from build123d import *

# Parameters (mm, degrees)
F2_R    = 1
F3_SIZE = 1


with BuildPart() as f1:
    # F0 (on Right) → F1 (revolve)
    with BuildSketch(Plane.YZ):
        Polygon((2.5, 27), (2.5, 0), (7.5, 0), (7.5, 30), (4, 30), (4, 50), (1.5, 50), (1.5, 27), align=None)
    revolve(axis=Axis((0, 0, 12.798217), (0, 0, -1)))

    # F2
    f2_edges = [f1.edges().sort_by_distance(p)[0] for p in [
        (0, -4, 50),
        (0, -4, 30),
        (0, -7.5, 30),
    ]]
    fillet(f2_edges, radius=F2_R)

    # F3
    f3_edges = [f1.edges().sort_by_distance(p)[0] for p in [
        (0, -7.5, 0),
    ]]
    chamfer(f3_edges, length=F3_SIZE)


solid = f1.part
The model under review builds one solid part; all positions refer to its coordinate system, in mm. A direction names the side the tool comes from. Give positions to 0.01 mm unless a question says otherwise; leave off trailing zeros. Write each loop counter-clockwise with the first axis right and the second up, starting at its lowest first coordinate (ties: lowest second). Pieces come first, ordered by that corner, then holes.
1. Tool access review of faces 1 (the flat face through (-1.3, 1.3, 50)), 2 (the flat face through (-5, 2, 30)): name each direction out of +Z, -Z, +X, -X, +Y, -Y from which nothing blocks a thin tool from reaching the whole face with its end or side.
2. Add section A-A, the plane y = 0. Write out the cut boundary in (x, z), plus the area to 3 significant figures.
3. Draft analysis for pull direction Y (two halves, no side actions). For faces 3 (the cylindrical face through (0.33, -7.493, 15.196)), 4 (the flat face through (0, -3, 0)), 5 (the flat face through (0, -2, 27)), 6 (the cylindrical face through (-2.44, -0.54, 13.31)), state which applies: +Y half, -Y half, draft (parallel to the pull), parting line (faces both ways), or undercut.
4. Wall thickness on L1, parallel to X at y = 0, z = 19.5; L2, parallel to X at y = 0, z = 33; L3, parallel to Y at x = -1.5, z = 26.5: over which ranges is each line inside the solid? List them lowest first.
5. For P1, Ø3, axis at x = -6, y = -4, coming from the -Z side; P2, Ø1, axis at y = 3.5, z = 42.5, coming from the -X side; P3, Ø3, axis at y = -5, z = 35.5, coming from the -X side; P4, Ø5, axis at x = -4.5, y = 5.5, coming from the +Z side, all flat-tipped, find the tip position at first contact; note any pin that passes through.
Worked answers:
1. face 1: +Z, +X, -X, +Y, -Y
1. face 2: +Z
2. outline: (-7.5, 1) - (-6.5, 0) - (-2.5, 0) - (-2.5, 27) - (-1.5, 27) - (-1.5, 50) - (-3, 50) arc R1 ccw to (-4, 49) - (-4, 31) arc R1 cw to (-5, 30) - (-6.5, 30) arc R1 ccw to (-7.5, 29) - close; (1.5, 27) - (2.5, 27) - (2.5, 0) - (6.5, 0) - (7.5, 1) - (7.5, 29) arc R1 ccw to (6.5, 30) - (5, 30) arc R1 cw to (4, 31) - (4, 49) arc R1 ccw to (3, 50) - (1.5, 50) - close
2. area: 405 mm2
3. face 3: parting line
3. face 4: draft
3. face 5: undercut
3. face 6: undercut
4. L1: x = -7.5 to -2.5, 2.5 to 7.5
4. L2: x = -4 to -1.5, 1.5 to 4
4. L3: y = -7.35 to -2, 2 to 7.35
5. P1: stops at z = 0
5. P2: stops at x = -2.65
5. P3: stops at x = -1.94
5. P4: stops at z = 30.08
